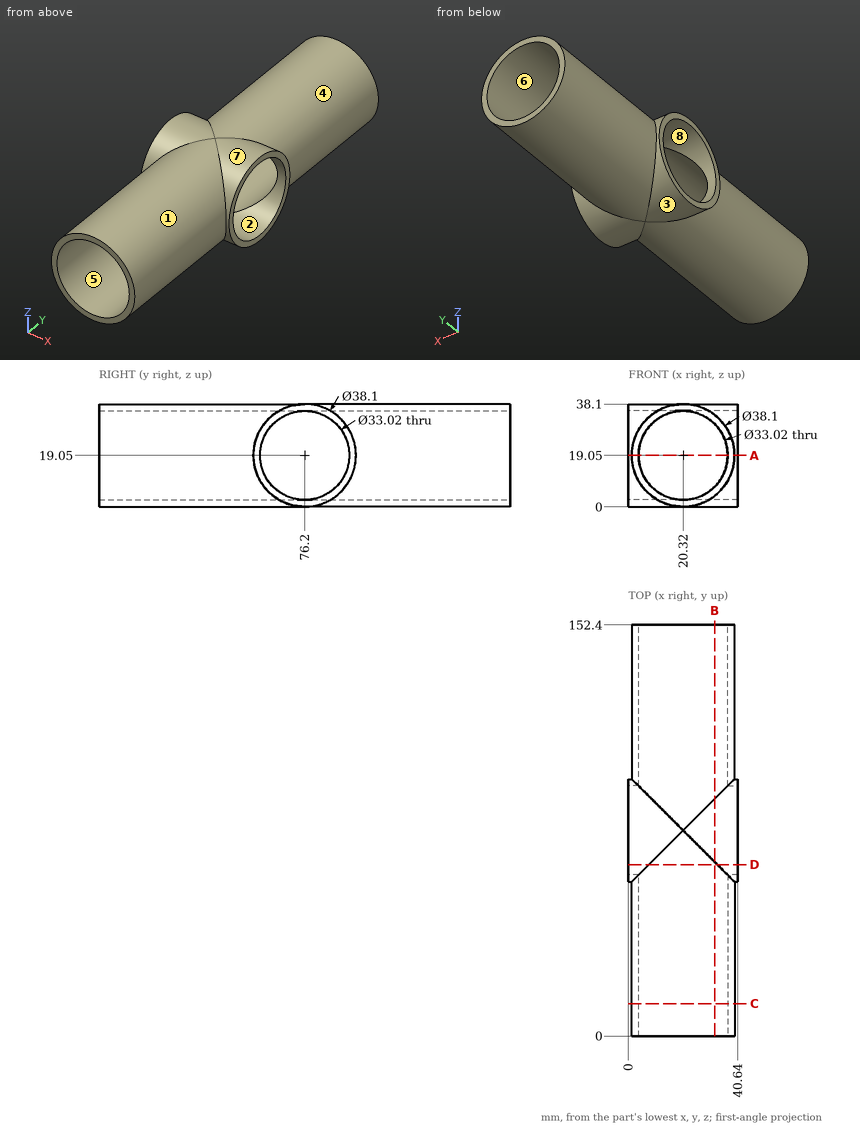
Job drawing, mm, ordinate dimensions from the low corner. One solid piece. A direction names the side the tool comes from. Give positions to 0.01 mm unless a question says otherwise; leave off trailing zeros. Loops run counter-clockwise (first coordinate to the right, second up) from the corner with the lowest first, then second, coordinate; pieces in that order, holes last. Notation, with made-up numbers: M 48,-1.5 L 66,-1.5 A20 cw 66,13.5 Z; hole C 41,-7.75 d6. An arc over 180 degrees is marked long. Use one line per item in the form item = value.
Item 1: Slice it at B-B on x = 32. List the corners of the cut face in (y, z), and give its area (3 significant figures).
Filled in:
outline = M 0,4 L 64.52,4 A19.05 ccw 87.88,4 L 152.4,4 L 152.4,7.38 L 87.88,7.38 A16.51 cw 64.52,7.38 L 0,7.38 Z; M 0,30.72 L 64.52,30.72 A16.51 cw 87.88,30.72 L 152.4,30.72 L 152.4,34.1 L 87.88,34.1 A19.05 ccw 64.52,34.1 L 0,34.1 Z
area = 1,000 mm^2
Item 2: Slice it at D-D on y = 63.5. List the corners of the cut face in (x, z).
Filled in:
outline = M 0,4.85 L 7.62,4.85 A19.05 ccw 33.02,4.85 L 40.64,4.85 L 40.64,8.5 L 33.02,8.5 A16.51 cw 7.62,8.5 L 0,8.5 Z; M 0,29.6 L 7.62,29.6 A16.51 cw 33.02,29.6 L 40.64,29.6 L 40.64,33.25 L 33.02,33.25 A19.05 ccw 7.62,33.25 L 0,33.25 Z
Item 3: Slice it at A-A on z = 19.05. List the corners of the cut face in (x, y).
Filled in:
outline = M 0,57.15 L 1.27,57.15 L 1.27,0 L 3.81,0 L 3.81,59.69 L 0,59.69 Z; M 0,92.71 L 3.81,92.71 L 3.81,152.4 L 1.27,152.4 L 1.27,95.25 L 0,95.25 Z; M 36.83,0 L 39.37,0 L 39.37,57.15 L 40.64,57.15 L 40.64,59.69 L 36.83,59.69 Z; M 36.83,92.71 L 40.64,92.71 L 40.64,95.25 L 39.37,95.25 L 39.37,152.4 L 36.83,152.4 Z
Item 4: Which spindle directions (+Z, -Z, +X, -X, +Y, -Y) get a long thin tool onto all of the face, cutting with end or side? Do the marked faces 1, 2, 3, 4 and 5. Say none if no direction does.
Filled in:
face_1 = -Y
face_2 = +X, -X
face_3 = -X
face_4 = +Y
face_5 = +Y, -Y
Item 5: Drill centre lines: L1, parallel to X at y = 12, z = 18.5; L2, parallel to Z at x = 5, y = 76.2; L3, parallel to X at y = 48, z = 25.5. Where is each one in solid material? Low to high.
Filled in:
L1 = 1.28 to 3.82, 36.82 to 39.36
L2 = 0 to 2.54, 35.56 to 38.1
L3 = 2.4 to 5.12, 35.52 to 38.24
Item 6: Flat gauge pins, fed straight in: pin 1 Ø3 at (x, y) = (13, 70) entering from -Z; pin 2 Ø2 at (y, z) = (121, 10) entering from -X; pin 3 Ø10 at (y, z) = (53.5, 29) entering from +X. Where does each tip first touch, or does it go through?
Filled in:
pin_1 = 0.59
pin_2 = 3.05
pin_3 = 38.72
Item 7: Two-plate mould, pull along Y, no slides. Class the marked faces 6, 7 and 8: released by +Y, released by -Y, zero draft, split by the parting line, or undercut.
Filled in:
face_6 = zero draft
face_7 = split by the parting line
face_8 = undercut
Item 8: Slice it at C-C on y = 12. List the corners of the cut face in (x, z).
Filled in:
outline = C 20.32,19.05 d38.1; hole C 20.32,19.05 d33.02
